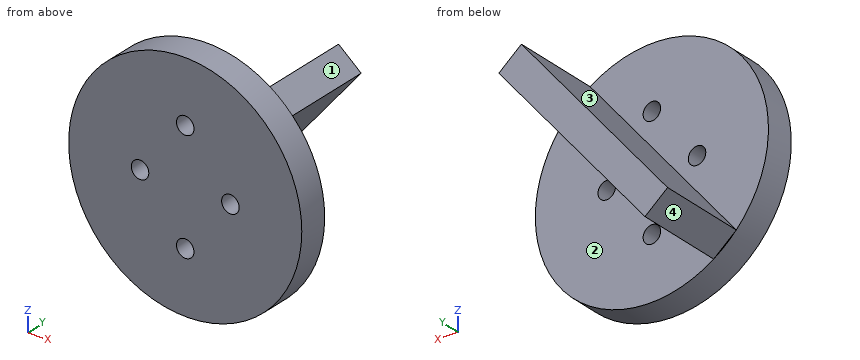
from build123d import *

# Parameters (mm, degrees)
SKETCH1_R           = 20
BOSS_EXTRUDE1_DEPTH = 5
CUT_EXTRUDE1_REACH  = 7
SKETCH2_R           = 1.5
BOSS_EXTRUDE2_DEPTH = 15


with BuildPart() as part:
    # Sketch1 → Boss-Extrude1 (new body)
    with BuildSketch(Plane(origin=(0, 0, 0), x_dir=(1, 0, 0), z_dir=(0, 1, 0))):
        Circle(SKETCH1_R)
    extrude(amount=BOSS_EXTRUDE1_DEPTH)

    # Sketch2 → Cut-Extrude1 (cut, up to next)
    with BuildSketch(Plane(origin=(0, 5, 0), x_dir=(1, 0, 0), z_dir=(0, 1, 0)), mode=Mode.PRIVATE) as cut_extrude1_sk1:
        with Locations((0, 9.5)):
            Circle(SKETCH2_R)
    cut_extrude1_tool1 = extrude(cut_extrude1_sk1.sketch, amount=-CUT_EXTRUDE1_REACH, mode=Mode.PRIVATE) & part.part
    add(cut_extrude1_tool1.solids().sort_by_distance((0, 5, -9.5))[0], mode=Mode.SUBTRACT)
    # Sketch2 → Cut-Extrude1 (cut, up to next)
    with BuildSketch(Plane(origin=(0, 5, 0), x_dir=(1, 0, 0), z_dir=(0, 1, 0)), mode=Mode.PRIVATE) as cut_extrude1_sk2:
        with Locations((0, -9.5)):
            Circle(SKETCH2_R)
    cut_extrude1_tool2 = extrude(cut_extrude1_sk2.sketch, amount=-CUT_EXTRUDE1_REACH, mode=Mode.PRIVATE) & part.part
    add(cut_extrude1_tool2.solids().sort_by_distance((0, 5, 9.5))[0], mode=Mode.SUBTRACT)
    # Sketch2 → Cut-Extrude1 (cut, up to next)
    with BuildSketch(Plane(origin=(0, 5, 0), x_dir=(1, 0, 0), z_dir=(0, 1, 0)), mode=Mode.PRIVATE) as cut_extrude1_sk3:
        with Locations((-7.75, 0)):
            Circle(SKETCH2_R)
    cut_extrude1_tool3 = extrude(cut_extrude1_sk3.sketch, amount=-CUT_EXTRUDE1_REACH, mode=Mode.PRIVATE) & part.part
    add(cut_extrude1_tool3.solids().sort_by_distance((-7.75, 5, 0))[0], mode=Mode.SUBTRACT)
    # Sketch2 → Cut-Extrude1 (cut, up to next)
    with BuildSketch(Plane(origin=(0, 5, 0), x_dir=(1, 0, 0), z_dir=(0, 1, 0)), mode=Mode.PRIVATE) as cut_extrude1_sk4:
        with Locations((7.75, 0)):
            Circle(SKETCH2_R)
    cut_extrude1_tool4 = extrude(cut_extrude1_sk4.sketch, amount=-CUT_EXTRUDE1_REACH, mode=Mode.PRIVATE) & part.part
    add(cut_extrude1_tool4.solids().sort_by_distance((7.75, 5, 0))[0], mode=Mode.SUBTRACT)

    # Sketch3 → Boss-Extrude2 (add)
    with BuildSketch(Plane(origin=(0, 5, 0), x_dir=(1, 0, 0), z_dir=(0, 1, 0))):
        Polygon((-14.480538437, 13.795434266), (10.606213333, -16.956067903), (14.480538437, -13.795434266), (-10.606213333, 16.956067903), align=None)
    extrude(amount=BOSS_EXTRUDE2_DEPTH)


solid = part.part
The listing builds one solid part. Answer for the finished solid, in the listing's coordinates (mm). Face numbers are marked on the shaded views. A direction names the side the tool comes from. Give positions to 0.01 mm unless a question says otherwise; leave off trailing zeros. Write each loop counter-clockwise with the first axis right and the second up, starting at its lowest first coordinate (ties: lowest second). Pieces come first, ordered by that corner, then holes.
1) Section B-B (y = 2.25) is taken. Write down the section's boundary in (x, z), and give its area (3 significant figures).
2) Given P1, Ø2, axis at y = 10, z = 4.5, coming from the +X side; P2, Ø5, axis at x = 7.75, z = 0, coming from the +Y side; P3, Ø2.5, axis at x = 0, z = -9.5, coming from the -Y side; P4, Ø10, axis at y = 11.5, z = -6, coming from the +X side, each flat-ended and moving along its own axis, determine where each tip first touches the part or whether it passes through.
3) Section D-D (x = 2) is taken. Write down the section's boundary in (y, z).
4) Section C-C (z = -9.5) is taken. Write down the section's boundary in (x, y).
5) Find the intervals of material crossed by L1, parallel to X at y = 3.15, z = 0; L2, parallel to Y at x = 9, z = -16; L3, parallel to X at y = 1.55, z = -9.5, in increasing order.
6) Section A-A (x = 8) is taken. Write down the section's boundary in (y, z).
7) A tool of negligible diameter and unlimited length cuts with its end or side. For the marked faces 1, 2, 3 and 4, from which of +Z, -Z, +X, -X, +Y, -Y can it reach the whole face along a straight path? Write none if from no direction.
Response:
1. outline: circle Ø40 at (0, 0); hole circle Ø3 at (-7.75, 0); hole circle Ø3 at (0, -9.5); hole circle Ø3 at (0, 9.5); hole circle Ø3 at (7.75, 0)
1. area: 1,230 mm2
2. P1: stops at x = 7.71
2. P2: stops at y = 5
2. P3: passes through
2. P4: stops at x = 2.41
3. outline: (0, -19.9) - (5, -19.9) - (5, -1.5) - (20, -1.5) - (20, 6.41) - (5, 6.41) - (5, 19.9) - (0, 19.9) - close
4. outline: (-17.6, 0) - (-1.5, 0) - (-1.5, 5) - (-4.52, 5) - (-4.52, 20) - (-10.98, 20) - (-10.98, 5) - (-17.6, 5) - close; (1.5, 0) - (17.6, 0) - (17.6, 5) - (1.5, 5) - close
5. L1: x = -20 to -9.25, -6.25 to 6.25, 9.25 to 20
5. L2: y = 0 to 5
5. L3: x = -17.6 to -1.5, 1.5 to 17.6
6. outline: (0, -18.33) - (5, -18.33) - (5, -1.48) - (0, -1.48) - close; (0, 1.48) - (5, 1.48) - (5, 5.85) - (20, 5.85) - (20, 13.76) - (5, 13.76) - (5, 18.33) - (0, 18.33) - close
7. face 1: +Z, +X, +Y
7. face 2: -Z, +X, +Y
7. face 3: +Z, -X, +Y
7. face 4: -Z, -X, +Y
